Input: part model. Units: mm. Frame: model coordinates. A direction names the side the tool comes from. Coordinates: 2 decimals unless noted, no trailing zeros. Write each loop counter-clockwise with the first axis right and the second up, starting at its lowest first coordinate (ties: lowest second). Pieces come first, ordered by that corner, then holes. Notation, with made-up numbers: (-8, 59) -> (32, 59) arc R25 cw to (32, 81) -> close; hole circle Ø10 at (80.5, 69). An arc over 180 degrees is marked (long way). Use one line per item in the form item = value. Start each with the question number.
(1) First-contact query: pin 1 (3 mm diameter, centred on x = 29.5, y = -5, fed in from +Z); pin 2 (1.6 mm diameter, centred on y = -2, z = -1.5, fed in from +X); pin 3 (0.7 mm diameter, centred on y = -2, z = -1.5, fed in from -X). Flat tips, straight axial feed; report the tip coordinate or a pass-through.
(2) Ray query, line 1 along Y through (x, z) = (4, 6); line 2 along Y through (x, z) = (81, -0.75); line 3 along X through (y, z) = (-9, -0.75). Return the intervals inside material, ascending.
(3) Set-up query: faces 1 (the face through (3.87, -24.12, 1.97)), 2 (the face through (93, -3, 7)), 3 (the face through (4.5, -15, -1)). Return all of +Z, -Z, +X, -X, +Y, -Y with unobstructed straight access to the full face (end or side cutting, diameter ignored); none if empty.
(4) Cut plane A-A on y = -12.5. Return the cut outline in (x, z).
(5) Cut plane D-D on y = -7.5. Return the cut outline in (x, z).
(6) Cut plane B-B on x = 17. Return the cut outline in (y, z).
(7) Cut plane C-C on z = 5. Return the cut outline in (x, y).
```python
from build123d import *

# Parameters (mm, degrees)
F1_DEPTH = 2
F3_R     = 3
F4_R     = 1
F2_R     = 2.5
F2_R_2   = 1.5
F5_DEPTH = 4
F6_DEPTH = 7


with BuildPart() as f1:
    # F0 (on Top) → F1 (new body)
    with BuildSketch(Plane.XY):
        Polygon((80, -3.433377482), (70, -3.433377482), (70, 0), (0, 0), (0, -30), (99, -30), (99, 0), (80, 0), align=None)
        with BuildLine():
            ThreePointArc((4.5, -11.5), (6.8431457505, -5.8431457505), (12.5, -3.5))
            Line((12.5, -3.5), (23, -3.5))
            ThreePointArc((23, -3.5), (28.6568542495, -5.8431457505), (31, -11.5))
            Line((31, -11.5), (31, -18.9))
            ThreePointArc((31, -18.9), (28.6568542495, -24.5568542495), (23, -26.9))
            Line((23, -26.9), (12.5, -26.9))
            ThreePointArc((12.5, -26.9), (6.8431457505, -24.5568542495), (4.5, -18.9))
            Line((4.5, -18.9), (4.5, -11.5))
        make_face(mode=Mode.SUBTRACT)
        with BuildLine():
            ThreePointArc((35.55, -11.5), (37.8931457505, -5.8431457505), (43.55, -3.5))
            Line((43.55, -3.5), (54.05, -3.5))
            ThreePointArc((54.05, -3.5), (59.7068542495, -5.8431457505), (62.05, -11.5))
            Line((62.05, -11.5), (62.05, -18.9))
            ThreePointArc((62.05, -18.9), (59.7068542495, -24.5568542495), (54.05, -26.9))
            Line((54.05, -26.9), (43.55, -26.9))
            ThreePointArc((43.55, -26.9), (37.8931457505, -24.5568542495), (35.55, -18.9))
            Line((35.55, -18.9), (35.55, -11.5))
        make_face(mode=Mode.SUBTRACT)
        with BuildLine():
            Line((84.5458595753, -3.5), (85.1, -3.5))
            ThreePointArc((85.1, -3.5), (90.7568542495, -5.8431457505), (93.1, -11.5))
            Line((93.1, -11.5), (93.1, -18.9))
            ThreePointArc((93.1, -18.9), (90.7568542495, -24.5568542495), (85.1, -26.9))
            Line((85.1, -26.9), (74.6, -26.9))
            ThreePointArc((74.6, -26.9), (68.9431457505, -24.5568542495), (66.6, -18.9))
            Line((66.6, -18.9), (66.6, -11.6456231289))
            ThreePointArc((66.6, -11.6456231289), (68.0644660941, -8.1100892229), (71.6, -6.6456231289))
            Line((71.6, -6.6456231289), (81.5458595753, -6.6456231289))
            ThreePointArc((81.5458595753, -6.6456231289), (82.6065197471, -6.2062833006), (83.0458595753, -5.1456231289))
            Line((83.0458595753, -5.1456231289), (83.0458595753, -5))
            ThreePointArc((83.0458595753, -5), (83.4851994035, -3.9393398282), (84.5458595753, -3.5))
        make_face(mode=Mode.SUBTRACT)
    extrude(amount=-F1_DEPTH)

    # F3
    f3_edges = [f1.edges().sort_by_distance(p)[0] for p in [
        (0, 0, -1),
        (0, -30, -1),
        (99, -30, -1),
        (99, 0, -1),
    ]]
    fillet(f3_edges, radius=F3_R)

    # F4
    f4_edges = [f1.edges().sort_by_distance(p)[0] for p in [
        (70, -3.433377, -1),
        (80, -3.433377, -1),
        (70, 0, -1),
        (80, 0, -1),
    ]]
    fillet(f4_edges, radius=F4_R)

    # F2 (on face) → F5 (join)
    with BuildSketch(Plane.XY):
        with Locations((4.2, -3.2)):
            Circle(F2_R)
        with Locations((4.2, -3.2)):
            Circle(F2_R_2, mode=Mode.SUBTRACT)
        with Locations((92.8, -3.2)):
            Circle(F2_R)
        with Locations((92.8, -3.2)):
            Circle(F2_R_2, mode=Mode.SUBTRACT)
        with Locations((92.8, -26.6)):
            Circle(F2_R)
        with Locations((92.8, -26.6)):
            Circle(F2_R_2, mode=Mode.SUBTRACT)
        with Locations((4.2, -26.6)):
            Circle(F2_R)
        with Locations((4.2, -26.6)):
            Circle(F2_R_2, mode=Mode.SUBTRACT)
    extrude(amount=F5_DEPTH)

    # F6 (add): faces of the model
    f6_faces = [f1.faces().sort_by_distance(p)[0] for p in [
        (4.2, -3.2, 0),
        (4.2, -26.6, 0),
        (92.8, -3.2, 0),
        (92.8, -26.6, 0),
    ]]
    extrude(f6_faces, amount=F6_DEPTH)


solid = f1.part
```
Values:
q1.pin_1 = 0
q1.pin_2 = 98.99
q1.pin_3 = 0.07
q2.line_1 = -28.09 to -25.11, -4.69 to -1.71
q2.line_2 = -30 to -26.9, -6.65 to 0
q2.line_3 = 0 to 4.9, 30.6 to 35.95, 61.65 to 67.36, 92.7 to 99
q3.face_1 = +Z
q3.face_2 = +Z, +X, -X, +Y, -Y
q3.face_3 = +Z, -Z
q4.outline = (0, -2) -> (4.5, -2) -> (4.5, 0) -> (0, 0) -> close; (31, -2) -> (35.55, -2) -> (35.55, 0) -> (31, 0) -> close; (62.05, -2) -> (66.6, -2) -> (66.6, 0) -> (62.05, 0) -> close; (93.1, -2) -> (99, -2) -> (99, 0) -> (93.1, 0) -> close
q5.outline = (0, -2) -> (5.57, -2) -> (5.57, 0) -> (0, 0) -> close; (29.93, -2) -> (36.62, -2) -> (36.62, 0) -> (29.93, 0) -> close; (60.98, -2) -> (68.8, -2) -> (68.8, 0) -> (60.98, 0) -> close; (92.03, -2) -> (99, -2) -> (99, 0) -> (92.03, 0) -> close
q6.outline = (-30, -2) -> (-26.9, -2) -> (-26.9, 0) -> (-30, 0) -> close; (-3.5, -2) -> (0, -2) -> (0, 0) -> (-3.5, 0) -> close
q7.outline = circle Ø3 at (4.2, -26.6); circle Ø3 at (4.2, -3.2); circle Ø3 at (92.8, -26.6); circle Ø3 at (92.8, -3.2)
